Autodesk Inventor part; units mm, degrees
ref_plane "YZ Plane" through (0, 0, 0) normal (1, 0, 0) x (0, 1, 0)
ref_plane "XZ Plane" through (0, 0, 0) normal (0, 1, 0) x (-1, 0, 0)
ref_plane "XY Plane" through (0, 0, 0) normal (0, 0, 1) x (1, 0, 0)
sketch "Sketch1" plane through (0, 0, 0) normal (0, 0, 1) x (1, 0, 0)
  line L0 (65, 8) -> (65, -5)
  line L1 (-5, -5) -> (-5, 8)
  line L2 (-5, 8) -> (65, 8)
  line L3 (65, 8) -> (65, -5)
  line L4 (65, -5) -> (-5, -5)
  line L5 (-5, 15) -> (65, 15)
  line L6 (65, 15) -> (65, -10)
  line L7 (65, -10) -> (-5, -10)
  line L8 (-5, -10) -> (-5, 15)
  line L9 (-5, 15) -> (65, -10) construction
  line L10 (65, 15) -> (-5, -10) construction
  point P0 (0, 0)
  point P1 (30, 2.5)
  dimension "d0" = 25
extrude "Extrusion1" add sketch "Sketch1" along normal blind 2.5
sketch "Sketch2" plane through (0, 0, 0) normal (0, 0, -1) x (-1, 0, 0)
  line L0 (-60, 0) -> (0, 0)
  line L1 (0, 0) -> (0, 3)
  line L2 (-60, 3) -> (0, 3)
  line L3 (-60, 0) -> (-60, 3)
  line L4 (0.35, -0.35) -> (-60.35, -0.35)
  line L5 (-60.35, -0.35) -> (-60.35, 3.35)
  line L6 (-60.35, 3.35) -> (0.35, 3.35)
  line L7 (0.35, 3.35) -> (0.35, -0.35)
  line L8 (-61.35, -1.35) -> (1.35, -1.35)
  line L9 (1.35, -1.35) -> (1.35, 4.35)
  line L10 (1.35, 4.35) -> (-61.35, 4.35)
  line L11 (-61.35, 4.35) -> (-61.35, -1.35)
  dimension "d3" = 0.35
  dimension "d4" = 1
extrude "Extrusion2" add sketch "Sketch2" along normal blind 5 contours L11 L10 L9 L8
fillet "Fillet1" radius 2 4 edges at (30, -1.35, 0) (-1.35, 1.5, 0) (30, 4.35, 0) (61.35, 1.5, 0)
sketch "Sketch3" plane through (0, 0, 0) normal (0, 0, -1) x (-1, 0, 0)
  line L0 (-65, -9.278) -> (-65, -5)
  line L1 (-47.2, 0) -> (-43.8, 0)
  line L2 (-45.5, 0) -> (-45.5, -10) construction
  line L3 (-16.2, 0) -> (-12.8, 0)
  line L4 (-14.5, 0) -> (-14.5, -7.5)
  circle A0 centre (-14.5, -7.5) radius 1.6
  line L5 (5, -10) -> (-65, -10) construction
  circle A1 centre (-14.5, -7.5) radius 1.5
  line L6 (-65, 2.5) -> (5, 2.5) construction
  line L7 (-65, -10) -> (-65, -5)
  line L8 (-65, -10) -> (-65, 15)
  line L9 (-65, -7.5) -> (5, -7.5) construction
  line L10 (5, 15) -> (5, -10) construction
  circle A2 centre (-45.5, -7.5) radius 1.6
  circle A3 centre (-14.5, 12.5) radius 1.6
  circle A4 centre (-45.5, 12.5) radius 1.6
  point P0 (0, 0)
  dimension "d11" = 3.2
  dimension "d28" = 3.2
extrude "Extrusion3" cut sketch "Sketch3" against normal up to surface (2.5 mm away) contours A1 | A0 | A2 | A3 | A4
sketch "Sketch4" plane through (0, 0, 2.5) normal (0, 0, 1) x (1, 0, 0)
  line L0 (65, -10) -> (65, 15)
  circle A0 centre (14.5, 12.5) radius 1.6
  circle A1 centre (45.5, -7.5) radius 1.6
  circle A2 centre (14.5, -7.5) radius 1.6
  circle A3 centre (45.5, 12.5) radius 1.6
  line L1 (-5, 15) -> (-5, -10)
  line L2 (-5, -10) -> (65, -10)
  line L3 (65, -10) -> (65, 15)
  line L4 (65, 15) -> (-5, 15)
  line L5 (65, 2.5) -> (-5, 2.5) construction
  line L6 (-5, 15) -> (-5, -10) construction
  line L7 (30, 15) -> (30, -10) construction
  line L8 (42.5, 27.5) -> (17.5, 27.5)
  line L9 (17.5, 27.5) -> (17.5, -22.5)
  line L10 (17.5, -22.5) -> (42.5, -22.5)
  line L11 (42.5, -22.5) -> (42.5, 27.5)
  line L12 (42.5, 27.5) -> (17.5, -22.5) construction
  line L13 (17.5, 27.5) -> (42.5, -22.5) construction
  circle A4 centre (39.5, -12.5) radius 1.6
  circle A5 centre (20.5, -12.5) radius 1.6
  circle A6 centre (39.5, 17.5) radius 1.6
  circle A7 centre (20.5, 17.5) radius 1.6
  point P0 (0, 0)
  point P1 (30, 2.5)
  point P2 (17.5, 15)
  point P3 (42.5, 15)
  point P4 (42.5, -10)
  point P5 (17.5, -10)
  dimension "d29" = 25
  dimension "d30" = 50
  dimension "d31" = 2.5
  dimension "d32" = 3
  dimension "d35" = 2.5
  dimension "d36" = 3
  dimension "d37" = 3.2
extrude "Extrusion4" add sketch "Sketch4" against normal up to surface (2.5 mm away) contours L11 L10 L9 L2 | L4 L9 L8 L11
fillet "Fillet2" radius 10 4 edges at (42.5, -10, 1.25) (42.5, 15, 1.25) (17.5, 15, 1.25) (17.5, -10, 1.25)
equation "\"d28\" = d11"
equation "\"d37\" = d11"
properties part number "CombineTestBase"
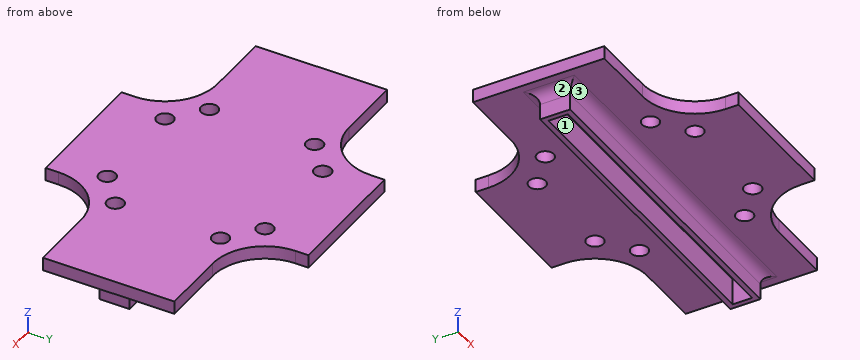
Geometry: final body of the model. Coordinates: model frame, mm. Face numbers are marked on the shaded views. Round coordinates to 2 decimals unless told otherwise and drop trailing zeros. Loops run counter-clockwise (first coordinate to the right, second up) from the corner with the lowest first, then second, coordinate; pieces in that order, holes last.
Q1. Pin query (flat end, axial travel): P1, Ø0.8, axis at y = -21.5, z = 2, coming from the -X side; P2, Ø0.8, axis at x = 58.5, z = 1.5, coming from the +Y side; P3, Ø2.5, axis at x = 45.5, y = -7.5, coming from the -Z side; P4, Ø5, axis at x = 45.5, y = 12.5, coming from the -Z side. Return the tip coordinate at first contact, or that it passes through.
Q2. Section C-C on z = 1.75. State how many separate pieces and enclosed holes the cut face has, plus the area to 3 significant figures.
Q3. Material intervals for L1, parallel to Y at x = 20.5, z = 1.45; L2, parallel to Y at x = 18, z = -1.75; L3, parallel to Y at x = 14.5, z = 1.55, sorted ascending.
Q4. Pull-direction query (X, two-part tool) for the marked faces 1, 2 and 3; classes: released by +X, released by -X, zero draft, split by the parting line, or undercut.
Q5. Section A-A on x = 20.5. Return loops of the section in (y, z).
Q6. Section B-B on y = 12.5. Return loops of the section in (x, z), plus the area to 3 significant figures.
Q7. Section D-D on z = -3. Return loops of the section in (x, y).
Evaluation:
1. P1: stops at x = 17.5
1. P2: stops at y = 15
1. P3: passes through
1. P4: stops at z = 0
2. separate pieces: 1
2. enclosed holes: 8
2. area: 2,400 mm2
3. L1: y = -22.5 to -14.1, -10.9 to 15.9, 19.1 to 27.5
3. L2: y = -1.37 to -0.35, 3.35 to 4.37
3. L3: y = -12.86 to -9.1, -5.9 to 10.9, 14.1 to 17.86
4. face 1: undercut
4. face 2: released by -X
4. face 3: zero draft
5. outline: (-22.5, 0) - (-14.1, 0) - (-14.1, 2.5) - (-22.5, 2.5) - close; (-10.9, 0) - (-3.35, 0) arc R2 cw to (-1.35, -2) - (-1.35, -5) - (-0.35, -5) - (-0.35, 0) - (3.35, 0) - (3.35, -5) - (4.35, -5) - (4.35, -2) arc R2 cw to (6.35, 0) - (15.9, 0) - (15.9, 2.5) - (-10.9, 2.5) - close; (19.1, 0) - (27.5, 0) - (27.5, 2.5) - (19.1, 2.5) - close
6. outline: (-5, 0) - (12.9, 0) - (12.9, 2.5) - (-5, 2.5) - close; (16.1, 0) - (43.9, 0) - (43.9, 2.5) - (16.1, 2.5) - close; (47.1, 0) - (65, 0) - (65, 2.5) - (47.1, 2.5) - close
6. area: 159 mm2
7. outline: (-1.35, -1.35) - (61.35, -1.35) - (61.35, 4.35) - (-1.35, 4.35) - close; hole (-0.35, -0.35) - (60.35, -0.35) - (60.35, 3.35) - (-0.35, 3.35) - close
